The model under review builds one solid part; all positions refer to its coordinate system, in mm. Coordinates: 2 decimals unless noted, no trailing zeros. Loops run counter-clockwise (first coordinate to the right, second up) from the corner with the lowest first, then second, coordinate; pieces in that order, holes last. Notation, with made-up numbers: (25, 45) - (57, 45) arc R22 cw to (57, 63) - close; hole circle Ø5 at (7, 57.25). An arc over 180 degrees is marked (long way). Use a Markdown table: item, result. Add a question column.
1) Add section A-A, the plane x = -37. Give the boundary of the cut face in (y, z), and give its area (3 significant figures).
2) Add section C-C, the plane y = -103.5. Give the boundary of the cut face in (x, z).
3) Add section B-B, the plane z = 1.3. Give the boundary of the cut face in (x, y), and give its area (3 significant figures).
4) Add section D-D, the plane x = 17. Give the boundary of the cut face in (y, z), and give its area (3 significant figures).
5) To check wall thickness, follow L1, parallel to Y at x = -16, z = 1.4; L2, parallel to X at y = -92, z = 1; L3, parallel to Y at x = -18, z = 0.7. State the ranges of each line that lie inside material, in increasing order. Write a range as [from, to].
6) Clearance check with flat-ended pins moving along their axes: pin 1 (1.8 mm diameter, centred on x = 7.61, y = -130.72, fed in from -Z); pin 2 (1 mm diameter, centred on y = -81.5, z = 0.5, fed in from -X); pin 3 (0.6 mm diameter, centred on y = -82, z = 1.5, fed in from +X). State where each tip first meets the part, or that it passes through.
```python
from build123d import *

# Parameters (mm, degrees)
SKETCH1_R           = 1.5
BOSS_EXTRUDE1_DEPTH = 2


with BuildPart() as part:
    # Sketch1 → Boss-Extrude1 (new body)
    with BuildSketch(Plane.XY):
        with BuildLine():
            Line((22.508911342, -130.69915726), (13.597675192, -130.983785211))
            Line((13.597675192, -130.983785211), (12.560733381, -127.954436921))
            ThreePointArc((12.560733381, -127.954436921), (12.064722619, -127.385308804), (11.312186404, -127.325119655))
            ThreePointArc((11.312186404, -127.325119655), (-26.483938318, -121.642871269), (-45.096768624, -88.26027792))
            Line((-45.096768624, -88.26027792), (-48.940455795, -84.8))
            Line((-48.940455795, -84.8), (-48.940455795, -79.8))
            Line((-48.940455795, -79.8), (-56.342527733, -79.8))
            Line((-56.342527733, -79.8), (-56.342527733, -84.8))
            ThreePointArc((-56.342527733, -84.8), (-34.007319131, -130.034150274), (15.867669408, -137.615404294))
            Line((15.867669408, -137.615404294), (14.673679255, -134.127250965))
            Line((14.673679255, -134.127250965), (22.749464344, -131.362920683))
            Line((22.749464344, -131.362920683), (22.508911342, -130.69915726))
        make_face()
        with Locations((7.607262335, -130.722795016)):
            Circle(SKETCH1_R, mode=Mode.SUBTRACT)
        with Locations((-37.543895432, -114.478381178)):
            Circle(SKETCH1_R, mode=Mode.SUBTRACT)
        with Locations((-47.172740285, -91.473829097)):
            Circle(SKETCH1_R, mode=Mode.SUBTRACT)
        with Locations((-17.271773957, -129.003020951)):
            Circle(SKETCH1_R, mode=Mode.SUBTRACT)
    extrude(amount=BOSS_EXTRUDE1_DEPTH)


solid = part.part
```
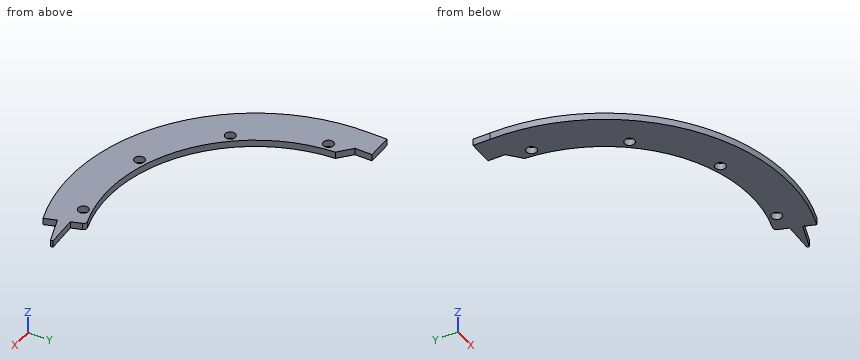
From the geometry:
| question | item | result |
|---|---|---|
| 1 | outline | (-127.68, 0) - (-115.88, 0) - (-115.88, 2) - (-127.68, 2) - close; (-113.08, 0) - (-111.31, 0) - (-111.31, 2) - (-113.08, 2) - close |
| 1 | area | 27.1 mm^2 |
| 2 | outline | (-53.47, 0) - (-41.47, 0) - (-41.47, 2) - (-53.47, 2) - close |
| 3 | outline | (-56.34, -84.8) arc R54.56 ccw to (15.87, -137.62) - (14.67, -134.13) - (22.75, -131.36) - (22.51, -130.7) - (13.6, -130.98) - (12.56, -127.95) arc R1 ccw to (11.31, -127.33) arc R43.36 cw to (-45.1, -88.26) - (-48.94, -84.8) - (-48.94, -79.8) - (-56.34, -79.8) - close; hole circle Ø3 at (-47.17, -91.47); hole circle Ø3 at (-37.54, -114.48); hole circle Ø3 at (-17.27, -129); hole circle Ø3 at (7.61, -130.72) |
| 3 | area | 1,070 mm^2 |
| 4 | outline | (-133.33, 0) - (-130.88, 0) - (-130.88, 2) - (-133.33, 2) - close |
| 4 | area | 4.91 mm^2 |
| 5 | L1 | y = [-138.68, -129.8], [-128.21, -126.96] |
| 5 | L2 | x = [-56.02, -48.58], [-45.77, -44.74] |
| 5 | L3 | y = [-138.09, -130.31], [-127.69, -126.22] |
| 6 | pin 1 | passes through |
| 6 | pin 2 | stops at x = -56.34 |
| 6 | pin 3 | stops at x = -48.94 |
